from build123d import *

# Parameters (mm, degrees)
BOSS_EXTRUDE1_DEPTH = 49.6
CUT_EXTRUDE1_REACH  = 74.214
SKETCH5_R           = 7
SKETCH5_W           = 12
SKETCH5_H           = 11
FILLET1_R           = 1


with BuildPart() as part:
    # Sketch4 → Boss-Extrude1 (new body)
    with BuildSketch(Plane.XY):
        Polygon((-50.9, 0), (50.9, 0), (52.4, -1.5), (50.9, -3), (-50.9, -3), (-52.4, -1.5), align=None)
    extrude(amount=BOSS_EXTRUDE1_DEPTH)

    # Sketch5 → Cut-Extrude1 (cut, up to next)
    with BuildSketch(Plane(origin=(0, 0, 0), x_dir=(1, 0, 0), z_dir=(0, 1, 0)), mode=Mode.PRIVATE) as cut_extrude1_sk1:
        with Locations(Location((-38.9, -15, 0), (0, 0, 180))):
            Circle(SKETCH5_R)
    cut_extrude1_tool1 = extrude(cut_extrude1_sk1.sketch, amount=-CUT_EXTRUDE1_REACH, mode=Mode.PRIVATE) & part.part
    # Sketch5 → Cut-Extrude1 (cut, up to next)
    with BuildSketch(Plane(origin=(0, 0, 0), x_dir=(1, 0, 0), z_dir=(0, 1, 0)), mode=Mode.PRIVATE) as cut_extrude1_sk2:
        with Locations((23.9, -15.5)):
            Rectangle(SKETCH5_W, SKETCH5_H)
    cut_extrude1_tool2 = extrude(cut_extrude1_sk2.sketch, amount=-CUT_EXTRUDE1_REACH, mode=Mode.PRIVATE) & part.part
    # Sketch5 → Cut-Extrude1 (cut, up to next)
    with BuildSketch(Plane(origin=(0, 0, 0), x_dir=(1, 0, 0), z_dir=(0, 1, 0)), mode=Mode.PRIVATE) as cut_extrude1_sk3:
        with BuildLine():
            Line((-15.9, -15), (-15.9, 0))
            Line((-15.9, 0), (-11.9, 0))
            Line((-11.9, 0), (-11.9, -20))
            Line((-11.9, -20), (-20.9, -20))
            ThreePointArc((-20.9, -20), (-24.435533906, -11.464466094), (-15.9, -15))
        make_face()
    cut_extrude1_tool3 = extrude(cut_extrude1_sk3.sketch, amount=-CUT_EXTRUDE1_REACH, mode=Mode.PRIVATE) & part.part
    # Sketch5 → Cut-Extrude1 (cut, up to next)
    with BuildSketch(Plane(origin=(0, 0, 0), x_dir=(1, 0, 0), z_dir=(0, 1, 0)), mode=Mode.PRIVATE) as cut_extrude1_sk4:
        with BuildLine():
            Line((-44.656064428, -42.593823795), (-44.656064428, -29.593823795))
            ThreePointArc((-44.656064428, -29.593823795), (-42.656064428, -27.593823795), (-40.656064428, -29.593823795))
            Line((-40.656064428, -29.593823795), (-40.656064428, -42.593823795))
            ThreePointArc((-40.656064428, -42.593823795), (-42.656064428, -44.593823795), (-44.656064428, -42.593823795))
        make_face()
    cut_extrude1_tool4 = extrude(cut_extrude1_sk4.sketch, amount=-CUT_EXTRUDE1_REACH, mode=Mode.PRIVATE) & part.part
    # Sketch5 → Cut-Extrude1 (cut, up to next)
    with BuildSketch(Plane(origin=(0, 0, 0), x_dir=(1, 0, 0), z_dir=(0, 1, 0)), mode=Mode.PRIVATE) as cut_extrude1_sk5:
        with BuildLine():
            Line((40.917781725, -42.593823795), (40.917781725, -7.593823795))
            ThreePointArc((40.917781725, -7.593823795), (42.917781725, -5.593823795), (44.917781725, -7.593823795))
            Line((44.917781725, -7.593823795), (44.917781725, -42.593823795))
            ThreePointArc((44.917781725, -42.593823795), (42.917781725, -44.593823795), (40.917781725, -42.593823795))
        make_face()
    cut_extrude1_tool5 = extrude(cut_extrude1_sk5.sketch, amount=-CUT_EXTRUDE1_REACH, mode=Mode.PRIVATE) & part.part
    # Sketch5 → Cut-Extrude1 (cut, up to next)
    with BuildSketch(Plane(origin=(0, 0, 0), x_dir=(1, 0, 0), z_dir=(0, 1, 0)), mode=Mode.PRIVATE) as cut_extrude1_sk6:
        with BuildLine():
            Line((-34.965522839, -42.593823795), (-34.965522839, -29.593823795))
            ThreePointArc((-34.965522839, -29.593823795), (-33.146064428, -27.774365385), (-31.326606018, -29.593823795))
            Line((-31.326606018, -29.593823795), (-31.326606018, -42.593823795))
            ThreePointArc((-31.326606018, -42.593823795), (-33.146064428, -44.413282206), (-34.965522839, -42.593823795))
        make_face()
    cut_extrude1_tool6 = extrude(cut_extrude1_sk6.sketch, amount=-CUT_EXTRUDE1_REACH, mode=Mode.PRIVATE) & part.part
    # Sketch5 → Cut-Extrude1 (cut, up to next)
    with BuildSketch(Plane(origin=(0, 0, 0), x_dir=(1, 0, 0), z_dir=(0, 1, 0)), mode=Mode.PRIVATE) as cut_extrude1_sk7:
        with BuildLine():
            Line((-25.457830531, -42.593823795), (-25.457830531, -29.593823795))
            ThreePointArc((-25.457830531, -29.593823795), (-23.638372121, -27.774365385), (-21.81891371, -29.593823795))
            Line((-21.81891371, -29.593823795), (-21.81891371, -42.593823795))
            ThreePointArc((-21.81891371, -42.593823795), (-23.638372121, -44.413282206), (-25.457830531, -42.593823795))
        make_face()
    cut_extrude1_tool7 = extrude(cut_extrude1_sk7.sketch, amount=-CUT_EXTRUDE1_REACH, mode=Mode.PRIVATE) & part.part
    # Sketch5 → Cut-Extrude1 (cut, up to next)
    with BuildSketch(Plane(origin=(0, 0, 0), x_dir=(1, 0, 0), z_dir=(0, 1, 0)), mode=Mode.PRIVATE) as cut_extrude1_sk8:
        with BuildLine():
            Line((-15.950138223, -42.593823795), (-15.950138223, -29.593823795))
            ThreePointArc((-15.950138223, -29.593823795), (-14.130679813, -27.774365385), (-12.311221403, -29.593823795))
            Line((-12.311221403, -29.593823795), (-12.311221403, -42.593823795))
            ThreePointArc((-12.311221403, -42.593823795), (-14.130679813, -44.413282206), (-15.950138223, -42.593823795))
        make_face()
    cut_extrude1_tool8 = extrude(cut_extrude1_sk8.sketch, amount=-CUT_EXTRUDE1_REACH, mode=Mode.PRIVATE) & part.part
    # Sketch5 → Cut-Extrude1 (cut, up to next)
    with BuildSketch(Plane(origin=(0, 0, 0), x_dir=(1, 0, 0), z_dir=(0, 1, 0)), mode=Mode.PRIVATE) as cut_extrude1_sk9:
        with BuildLine():
            Line((-6.622987505, -42.593823795), (-6.622987505, -7.593823795))
            ThreePointArc((-6.622987505, -7.593823795), (-4.622987505, -5.593823795), (-2.622987505, -7.593823795))
            Line((-2.622987505, -7.593823795), (-2.622987505, -42.593823795))
            ThreePointArc((-2.622987505, -42.593823795), (-4.622987505, -44.593823795), (-6.622987505, -42.593823795))
        make_face()
    cut_extrude1_tool9 = extrude(cut_extrude1_sk9.sketch, amount=-CUT_EXTRUDE1_REACH, mode=Mode.PRIVATE) & part.part
    # Sketch5 → Cut-Extrude1 (cut, up to next)
    with BuildSketch(Plane(origin=(0, 0, 0), x_dir=(1, 0, 0), z_dir=(0, 1, 0)), mode=Mode.PRIVATE) as cut_extrude1_sk10:
        with BuildLine():
            Line((2.884704802, -42.593823795), (2.884704802, -7.593823795))
            ThreePointArc((2.884704802, -7.593823795), (4.884704802, -5.593823795), (6.884704802, -7.593823795))
            Line((6.884704802, -7.593823795), (6.884704802, -42.593823795))
            ThreePointArc((6.884704802, -42.593823795), (4.884704802, -44.593823795), (2.884704802, -42.593823795))
        make_face()
    cut_extrude1_tool10 = extrude(cut_extrude1_sk10.sketch, amount=-CUT_EXTRUDE1_REACH, mode=Mode.PRIVATE) & part.part
    # Sketch5 → Cut-Extrude1 (cut, up to next)
    with BuildSketch(Plane(origin=(0, 0, 0), x_dir=(1, 0, 0), z_dir=(0, 1, 0)), mode=Mode.PRIVATE) as cut_extrude1_sk11:
        with BuildLine():
            Line((12.5729387, -42.593823795), (12.5729387, -29.593823795))
            ThreePointArc((12.5729387, -29.593823795), (14.39239711, -27.774365385), (16.211855521, -29.593823795))
            Line((16.211855521, -29.593823795), (16.211855521, -42.593823795))
            ThreePointArc((16.211855521, -42.593823795), (14.39239711, -44.413282206), (12.5729387, -42.593823795))
        make_face()
    cut_extrude1_tool11 = extrude(cut_extrude1_sk11.sketch, amount=-CUT_EXTRUDE1_REACH, mode=Mode.PRIVATE) & part.part
    # Sketch5 → Cut-Extrude1 (cut, up to next)
    with BuildSketch(Plane(origin=(0, 0, 0), x_dir=(1, 0, 0), z_dir=(0, 1, 0)), mode=Mode.PRIVATE) as cut_extrude1_sk12:
        with BuildLine():
            Line((22.080631007, -42.593823795), (22.080631007, -29.593823795))
            ThreePointArc((22.080631007, -29.593823795), (23.900089418, -27.774365385), (25.719547828, -29.593823795))
            Line((25.719547828, -29.593823795), (25.719547828, -42.593823795))
            ThreePointArc((25.719547828, -42.593823795), (23.900089418, -44.413282206), (22.080631007, -42.593823795))
        make_face()
    cut_extrude1_tool12 = extrude(cut_extrude1_sk12.sketch, amount=-CUT_EXTRUDE1_REACH, mode=Mode.PRIVATE) & part.part
    # Sketch5 → Cut-Extrude1 (cut, up to next)
    with BuildSketch(Plane(origin=(0, 0, 0), x_dir=(1, 0, 0), z_dir=(0, 1, 0)), mode=Mode.PRIVATE) as cut_extrude1_sk13:
        with BuildLine():
            Line((31.588323315, -42.593823795), (31.588323315, -29.593823795))
            ThreePointArc((31.588323315, -29.593823795), (33.407781725, -27.774365385), (35.227240136, -29.593823795))
            Line((35.227240136, -29.593823795), (35.227240136, -42.593823795))
            ThreePointArc((35.227240136, -42.593823795), (33.407781725, -44.413282206), (31.588323315, -42.593823795))
        make_face()
    cut_extrude1_tool13 = extrude(cut_extrude1_sk13.sketch, amount=-CUT_EXTRUDE1_REACH, mode=Mode.PRIVATE) & part.part
    add(cut_extrude1_tool1.solids().sort_by_distance((-38.9, 0, 15))[0], mode=Mode.SUBTRACT)
    add(cut_extrude1_tool2.solids().sort_by_distance((23.9, 0, 15.5))[0], mode=Mode.SUBTRACT)
    add(cut_extrude1_tool3.solids().sort_by_distance((-17.356278, 0, 12.686666))[0], mode=Mode.SUBTRACT)
    add(cut_extrude1_tool4.solids().sort_by_distance((-42.656064, 0, 36.093824))[0], mode=Mode.SUBTRACT)
    add(cut_extrude1_tool5.solids().sort_by_distance((42.917782, 0, 25.093824))[0], mode=Mode.SUBTRACT)
    add(cut_extrude1_tool6.solids().sort_by_distance((-33.146064, 0, 36.093824))[0], mode=Mode.SUBTRACT)
    add(cut_extrude1_tool7.solids().sort_by_distance((-23.638372, 0, 36.093824))[0], mode=Mode.SUBTRACT)
    add(cut_extrude1_tool8.solids().sort_by_distance((-14.13068, 0, 36.093824))[0], mode=Mode.SUBTRACT)
    add(cut_extrude1_tool9.solids().sort_by_distance((-4.622988, 0, 25.093824))[0], mode=Mode.SUBTRACT)
    add(cut_extrude1_tool10.solids().sort_by_distance((4.884705, 0, 25.093824))[0], mode=Mode.SUBTRACT)
    add(cut_extrude1_tool11.solids().sort_by_distance((14.392397, 0, 36.093824))[0], mode=Mode.SUBTRACT)
    add(cut_extrude1_tool12.solids().sort_by_distance((23.900089, 0, 36.093824))[0], mode=Mode.SUBTRACT)
    add(cut_extrude1_tool13.solids().sort_by_distance((33.407782, 0, 36.093824))[0], mode=Mode.SUBTRACT)

    # Fillet1
    fillet1_edges = [part.edges().sort_by_distance(p)[0] for p in [
        (-11.9, -1.5, 20),
    ]]
    fillet(fillet1_edges, radius=FILLET1_R)
    fillet1_2_edges = [part.edges().sort_by_distance(p)[0] for p in [
        (-15.9, -1.5, 15),
    ]]
    fillet(fillet1_2_edges, radius=FILLET1_R)


solid = part.part
The model under review builds one solid part; all positions refer to its coordinate system, in mm. A direction names the side the tool comes from. Give positions to 0.01 mm unless a question says otherwise; leave off trailing zeros. Loops run counter-clockwise (first coordinate to the right, second up) from the corner with the lowest first, then second, coordinate; pieces in that order, holes last. Notation, with made-up numbers: (-5.75, 46) -> (16.25, 46) arc R13 cw to (16.25, 52) -> close; hole circle Ø11 at (75, 36.5). An arc over 180 degrees is marked (long way). Answer as a JSON object with one key per item and string values. Group by question number.
Q1. Tool access review of faces 1 (the flat face through (-1, 0, 24)), 2 (the flat face through (-34.966, -1, 36)): name each direction out of +Z, -Z, +X, -X, +Y, -Y from which nothing blocks a thin tool from reaching the whole face with its end or side.
Q2. Take a section at D-D (x = 5). Write out the cut boundary in (y, z), plus the area to 3 significant figures.
Q3. Insertion check: pin 1 (0.9 mm diameter, centred on y = -1, z = 28, fed in from -X); pin 2 (0.9 mm diameter, centred on y = -2, z = 39, fed in from +X); pin 3 (11 mm diameter, centred on x = -38.9, z = 15, fed in from -Y). Each pin has a flat end and moves straight along its axis. Give the tip position at first contact, or say it passes through.
Q4. Take a section at A-A (z = 15). State how many separate pieces and enclosed holes the cut face has, plus the area to 3 significant figures.
Q5. Draft analysis for pull direction X (two halves, no side actions). For faces 3 (the flat face through (-34, -1, 0)), 4 (the cylindrical face through (-42.612, -1.479, 44.593)), 5 (the flat face through (-25.458, -1, 36)), state which applies: pulls with the +X half, pulls with the -X half, needs draft (parallel to the pull), parting line crosses it, or undercut.
Q6. Take a section at B-B (x = -38.9). Write out the cut boundary in (y, z).
Q7. Wall thickness on line 1 along Z through (x, y) = (-20.9, -1.95); line 2 along Z through (x, y) = (-34, -0.7); line 3 along Z through (x, y) = (-38.9, -1.4): over which ranges is each line inside the solid? List them lowest first.
Answer below:
{
 "1": {"face 1": "+Z, -Z, +X, -X, +Y", "face 2": "+Y, -Y"},
 "2": {"outline": "(-3, 0) -> (0, 0) -> (0, 5.6) -> (-3, 5.6) -> close; (-3, 44.59) -> (0, 44.59) -> (0, 49.6) -> (-3, 49.6) -> close", "area": "31.8 mm2"},
 "3": {"pin 1": "stops at x = -52.35", "pin 2": "stops at x = 52.35", "pin 3": "passes through"},
 "4": {"separate pieces": "7", "enclosed holes": "0", "area": "154 mm2"},
 "5": {"face 3": "needs draft", "face 4": "undercut", "face 5": "undercut"},
 "6": {"outline": "(-3, 0) -> (0, 0) -> (0, 8) -> (-3, 8) -> close; (-3, 22) -> (0, 22) -> (0, 49.6) -> (-3, 49.6) -> close"},
 "7": {"line 1": "z = 0 to 10, 20 to 49.6", "line 2": "z = 0 to 10, 20 to 27.99, 44.2 to 49.6", "line 3": "z = 0 to 8, 22 to 49.6"}
}
